from build123d import *

# Parameters (mm, degrees)
SKETCH_1_W          = 89.675670072
SKETCH_1_H          = 82.296703234
EXTRUDE_1_DEPTH     = 10
SKETCH_3_R          = 6
CUT_EXTRUDE_1_DEPTH = 2
SKETCH_4_R          = 6
CUT_EXTRUDE_2_DEPTH = 2


with BuildPart() as part:
    # Sketch 1 → Extrude 1 (new body)
    with BuildSketch(Plane.XY):
        Rectangle(SKETCH_1_W, SKETCH_1_H)
    extrude(amount=EXTRUDE_1_DEPTH)

    # Sketch 3 → Cut-Extrude 1 (cut)
    with BuildSketch(Plane.XY.offset(10)):
        with Locations((-30.411848961, 30.989289131)):
            Circle(SKETCH_3_R)
        with Locations(Location((30.411848961, 30.989289131, 0), (0, 0, 180))):
            Circle(SKETCH_3_R)
    extrude(amount=-CUT_EXTRUDE_1_DEPTH, mode=Mode.SUBTRACT)

    # Sketch 4 → Cut-Extrude 2 (cut)
    with BuildSketch(Plane.XY.offset(10)):
        with Locations((0, 30.989289131)):
            Circle(SKETCH_4_R)
    extrude(amount=-CUT_EXTRUDE_2_DEPTH, mode=Mode.SUBTRACT)


solid = part.part
Geometry check sheet. Reference: the model listing, model coordinates, mm. A direction names the side the tool comes from. Coordinates: 2 decimals unless noted, no trailing zeros. Order: outer loops, then holes, each group sorted by start corner. A loop starts at its lowest first (then second) coordinate and runs counter-clockwise, first axis right, second up. Notation, with made-up numbers: (-29.5, -21.75) - (-6.5, -21.75) arc R3 cw to (-6.5, -17.75) - close; hole circle Ø11 at (-23.75, 26.5). An arc over 180 degrees is marked (long way). Answer in a Markdown table with one row per item. Add a question column.
1) Cross-section at B-B, the plane x = -29. Record the cut outline in (y, z).
2) Material ranges on line 1 along Y through (x, z) = (0, 9.2); line 2 along Z through (x, y) = (26, 35); line 3 along Y through (x, z) = (35, 8.75), recorded low to high. Write a range as [from, to].
3) Gauge pin test, flat ends, axial feed: P1, Ø3, axis at x = -25, y = 2, coming from the -Z side; P2, Ø3.5, axis at x = -30, y = 31.5, coming from the +Z side. Record the tip position at first contact, or that the pin passes through.
4) Set-up check for faces 4 (the flat face through (0, 31, 8)), 5 (the flat face through (-1, 41.148, 5)): record each of +Z, -Z, +X, -X, +Y, -Y from which the full face is reachable in a straight line by a thin tool's end or side.
5) Release check for a two-part mould opening along X. For faces 1 (the flat face through (-44.838, -1, 5)), 2 (the cylindrical face through (34.8, 26.9, 9)), 3 (the flat face through (-1, 1, 0)) record: +X half, -X half, draft (parallel to the pull), parting line (faces both ways), or undercut.
6) Cross-section at A-A, the plane x = 0. Record the cut outline in (y, z), then the cut area to 3 significant figures.
Check result:
| question | item | result |
|---|---|---|
| 1 | outline | (-41.15, 0) - (41.15, 0) - (41.15, 10) - (36.82, 10) - (36.82, 8) - (25.16, 8) - (25.16, 10) - (-41.15, 10) - close |
| 2 | line 1 | y = [-41.15, 24.99], [36.99, 41.15] |
| 2 | line 2 | z = [0, 8] |
| 2 | line 3 | y = [-41.15, 27.12], [34.86, 41.15] |
| 3 | P1 | stops at z = 0 |
| 3 | P2 | stops at z = 8 |
| 4 | face 4 | +Z |
| 4 | face 5 | +Z, -Z, +X, -X, +Y |
| 5 | face 1 | -X half |
| 5 | face 2 | undercut |
| 5 | face 3 | draft |
| 6 | outline | (-41.15, 0) - (41.15, 0) - (41.15, 10) - (36.99, 10) - (36.99, 8) - (24.99, 8) - (24.99, 10) - (-41.15, 10) - close |
| 6 | area | 799 mm² |
